Source: three-view drawing plus pictorial views. Frame: mm from the lowest corner of the part. A direction names the side the tool comes from. Coordinates: 2 decimals unless noted, no trailing zeros. Order: outer loops, then holes, each group sorted by start corner. A loop starts at its lowest first (then second) coordinate and runs counter-clockwise, first axis right, second up. Notation, with made-up numbers: M 44,60 L 88,60 A29 cw 88,93 Z; hole C 16.25,87 d11. An arc over 180 degrees is marked long. One line per question, with ' | ' between items.
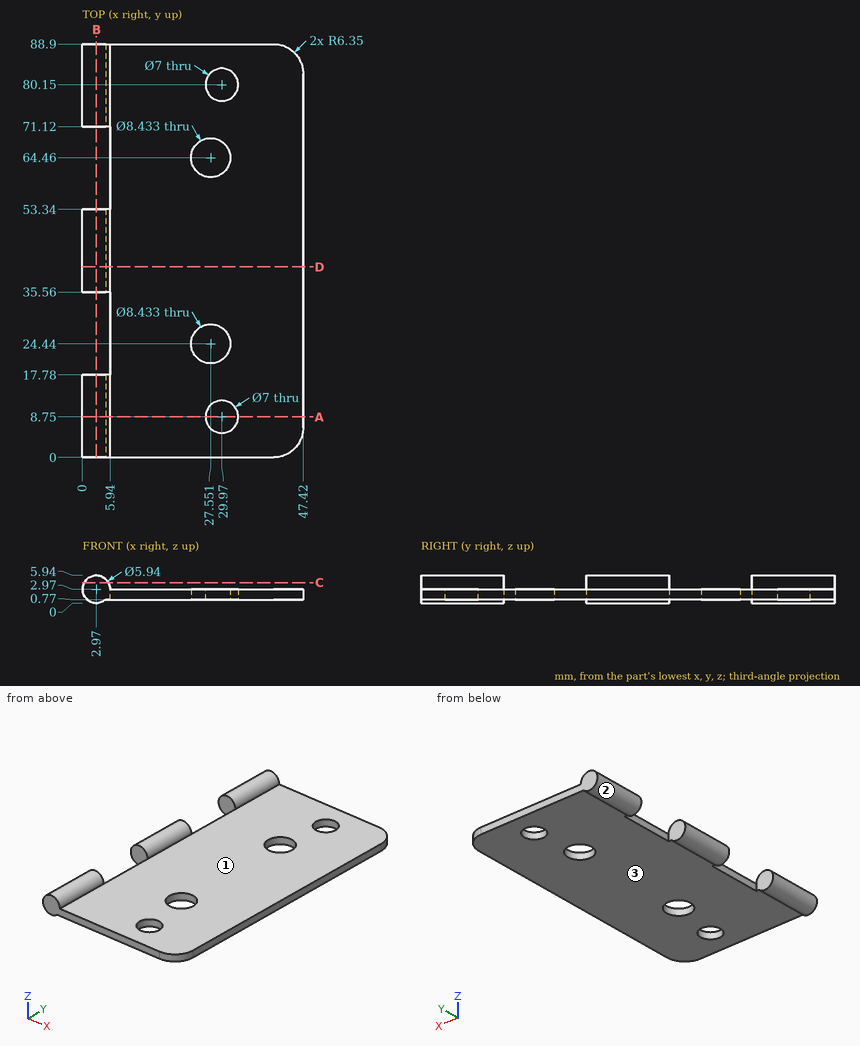
1. Pin query (flat end, axial travel): P1, Ø8, axis at x = 29.97, y = 8.75, coming from the -Z side; P2, Ø1.5, axis at x = 36.5, y = 51, coming from the +Z side; P3, Ø1.1, axis at y = 25.5, z = 2, coming from the -X side. Return the tip coordinate at first contact, or that it passes through.
Response values:
P1: stops at z = 0.77 | P2: stops at z = 2.97 | P3: stops at x = 5.94
2. Section C-C, the plane z = 4.4. Output: boundary loops of the cut face in (x, y), and give its area (3 significant figures).
Response values:
outline: M 0.37,0 L 5.57,0 L 5.57,17.78 L 0.37,17.78 Z; M 0.37,35.56 L 5.57,35.56 L 5.57,53.34 L 0.37,53.34 Z; M 0.37,71.12 L 5.57,71.12 L 5.57,88.9 L 0.37,88.9 Z | area: 278 mm^2
3. Access query for the marked faces 1, 2 and 3. Directions: +Z, -Z, +X, -X, +Y, -Y. A direction counts if a zero-diameter tool reaches every point of the face in a straight line with its end or side. Return the directions, or none.
Response values:
face 1: +Z, +X, +Y, -Y | face 2: +Y, -Y | face 3: -Z, +X, +Y, -Y
4. Section B-B, the plane x = 2.97. Output: boundary loops of the cut face in (y, z), and give its area (3 significant figures).
Response values:
outline: M 0,0 L 17.78,0 L 17.78,5.94 L 0,5.94 Z; M 35.56,0 L 53.34,0 L 53.34,5.94 L 35.56,5.94 Z; M 71.12,0 L 88.9,0 L 88.9,5.94 L 71.12,5.94 Z | area: 317 mm^2
5. Section D-D, the plane y = 41. Output: boundary loops of the cut face in (x, z) (1 decimal).
Response values:
outline: M 5,0.8 L 47.4,0.8 L 47.4,3 L 5.9,3 A3 ccw long Z
6. Section A-A, the plane y = 8.75. Output: boundary loops of the cut face in (x, z) (1 decimal).
Response values:
outline: M 5,0.8 L 26.5,0.8 L 26.5,3 L 5.9,3 A3 ccw long Z; M 33.5,0.8 L 47.4,0.8 L 47.4,3 L 33.5,3 Z
7. Material intervals for line 1 (X direction, y = 55, z = 1.15); line 2 (Z direction, x = 43, y = 77); line 3 (X direction, y = 9, z = 1.3) (1 decimal), sorted ascending. Write a range as [from, to].
Response values:
line 1: x = [5.94, 47.42] | line 2: z = [0.77, 2.97] | line 3: x = [0.5, 26.5], [33.5, 47.4]
